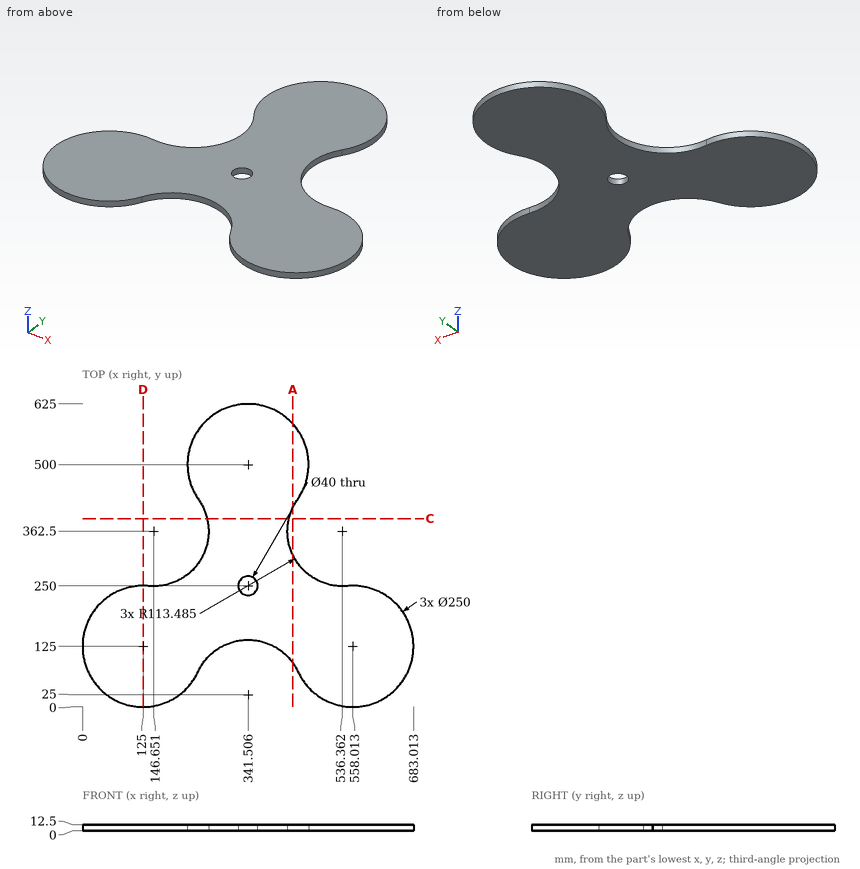
Here's the drawing with two shaded views (mm, measured from the low corner). I have some questions. Round coordinates to 2 decimals unless told otherwise and drop trailing zeros. Loops run counter-clockwise (first coordinate to the right, second up) from the corner with the lowest first, then second, coordinate; pieces in that order, holes last.
Item 1: Please list where these lines run through material, in increasing order: L1, parallel to Y at x = 236.5, z = 2.75 (1 decimal); L2, parallel to Y at x = 375.5, z = 3.5 (1 decimal); L3, parallel to X at y = 455, z = 3 (1 decimal).
Item 2: Suppose I cut it at C-C, the plane y = 388.5. Write out the boundary of the cut face in (x, z), then the cut area to 3 significant figures.
Item 3: Will these pins go through, and if not, where does the flat tip stop? pin 1 Ø3 at (x, z) = (145.5, 7) entering from +Y; pin 2 Ø6 at (y, z) = (320, 7.5) entering from +X; pin 3 Ø5 at (x, z) = (433.5, 8) entering from +Y; pin 4 Ø10 at (x, y) = (113.5, 230.5) entering from -Z.
Item 4: Suppose I cut it at A-A, the plane x = 434. Write out the boundary of the cut face in (y, z) (1 decimal).
Item 5: Suppose I cut it at D-D, the plane x = 125. Write out the boundary of the cut face in (y, z), then the cut area to 4 significant figures.
Reported:
1. L1: y = 68.5 to 293.2, 432.2 to 567.8
1. L2: y = 133.3 to 620.3
1. L3: x = 224.9 to 458.1
2. outline: (257.12, 0) - (425.9, 0) - (425.9, 12.5) - (257.12, 12.5) - close
2. area: 2,110 mm2
3. pin 1: stops at y = 249.05
3. pin 2: stops at x = 432.4
3. pin 3: stops at y = 587.27
3. pin 4: stops at z = 0
4. outline: (90.8, 0) - (313.5, 0) - (313.5, 12.5) - (90.8, 12.5) - close; (411.5, 0) - (584.1, 0) - (584.1, 12.5) - (411.5, 12.5) - close
5. outline: (0, 0) - (250, 0) - (250, 12.5) - (0, 12.5) - close
5. area: 3,125 mm2
